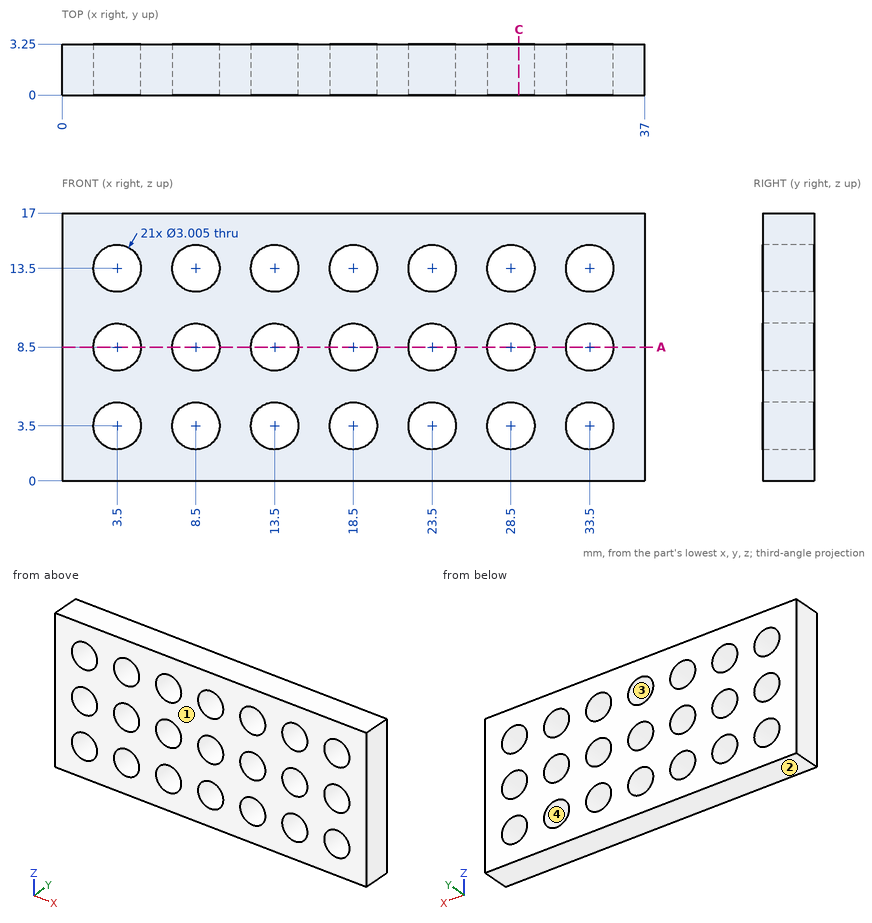
Print and shaded views of the part. All mm, measured from the part's lowest x, y and z. Round coordinates to 2 decimals unless told otherwise and drop trailing zeros. Loops run counter-clockwise (first coordinate to the right, second up) from the corner with the lowest first, then second, coordinate; pieces in that order, holes last. Notation, with made-up numbers: (-38, 32) -> (8, 32) arc R27 cw to (8, 65) -> close; hole circle Ø11 at (-17.75, -24.5). An arc over 180 degrees is marked (long way). Use CSV: the item, a comma, the result in double quotes. Start each with the question number.
1) Cut at A-A, the plane z = 8.5. Give the number of separate pieces and of enclosed holes in the cut face, plus the area to 3 significant figures.
2) Wall check: L1, parallel to Z at x = 18.5, y = 1.45; L2, parallel to Z at x = 7.5, y = 2.2. Give the ranges that are in metal, low to high. Write a range as [from, to].
3) Drop a flat-ended pin along its axis: P1, Ø3.5, axis at x = 8.5, z = 13.5, coming from the +Y side. Give the stop position or say it passes through.
4) Cut at C-C, the plane x = 29. Write the cut outline in (y, z).
5) Pull direction Z, two halves, no side cores. Call the marked faces 1, 2, 3 and 4: +Z half, -Z half, draft (parallel to the pull), parting line (faces both ways), or undercut.
Determined:
1,separate pieces,"8"
1,enclosed holes,"0"
1,area,"51.9 mm2"
2,L1,"z = [0, 2], [5, 7], [10, 12], [15, 17]"
2,L2,"z = [0, 2.38], [4.62, 7.38], [9.62, 12.38], [14.62, 17]"
3,P1,"stops at y = 3.25"
4,outline,"(0, 0) -> (3.25, 0) -> (3.25, 2.08) -> (0, 2.08) -> close; (0, 4.92) -> (3.25, 4.92) -> (3.25, 7.08) -> (0, 7.08) -> close; (0, 9.92) -> (3.25, 9.92) -> (3.25, 12.08) -> (0, 12.08) -> close; (0, 14.92) -> (3.25, 14.92) -> (3.25, 17) -> (0, 17) -> close"
5,face 1,"draft"
5,face 2,"-Z half"
5,face 3,"undercut"
5,face 4,"undercut"
